Can you work these out from the model? Positions are in its coordinate system, mm. Round coordinates to 2 decimals unless told otherwise and drop trailing zeros. Write each loop counter-clockwise with the first axis right and the second up, starting at its lowest first coordinate (ties: lowest second). Pieces come first, ordered by that corner, then holes. Notation, with made-up numbers: M 22.5,66.25 L 59.5,66.25 A16 cw 59.5,91.25 Z; hole C -6,70 d11. An arc over 180 degrees is marked long. Answer as a JSON object with one key per item and string values. Group by question number.
1) Please list where these lines run through material, in increasing order: L1, parallel to X at y = 1.75, z = 54; L2, parallel to Z at x = 16, y = 1.6; L3, parallel to Z at x = -10.5, y = 0.4. Write a range as [from, to].
2) Suppose I cut it at A-A, the plane x = 24. State how many separate pieces and enclosed holes the cut face has, and give its area (3 significant figures).
3) I'm going to push flat-ended pins straight in: pin 1 Ø1 at (x, y) = (8, 0.5) entering from -Z; pin 2 Ø0.6 at (x, y) = (26, 0.5) entering from -Z; pin 3 Ø8 at (x, z) = (-10, 19) entering from -Y. Where does each tip first touch, or does it pass through?
4) Suppose I cut it at B-B, the plane z = 22. Write out the boundary of the cut face in (x, y).
from build123d import *

# Parameters (mm, degrees)
SKETCH2_W           = 105
SKETCH2_H           = 69
SKETCH2_W_2         = 12.176237233
SKETCH2_H_2         = 12
SKETCH2_W_3         = 12
SKETCH2_W_4         = 11
SKETCH2_H_3         = 11
SKETCH2_W_5         = 10.781198293
BOSS_EXTRUDE1_DEPTH = 2
FILLET1_R           = 5
FILLET2_R           = 5
CHAMFER1_SIZE       = 2
SKETCH3_W           = 12.4
SKETCH3_H           = 12.584292926
SKETCH3_W_2         = 12.5
SKETCH3_W_3         = 12.6
SKETCH3_W_4         = 12.2
SKETCH3_H_2         = 12.9
SKETCH3_H_3         = 12.6
CUT_EXTRUDE1_DEPTH  = 10
SKETCH4_W           = 0.6
SKETCH4_H           = 11
BOSS_EXTRUDE2_DEPTH = 2
SKETCH5_W           = 0.6
SKETCH5_H           = 11
BOSS_EXTRUDE3_DEPTH = 2
SKETCH6_W           = 0.8
SKETCH6_H           = 11
SKETCH6_W_2         = 0.4
SKETCH6_W_3         = 0.776237233
BOSS_EXTRUDE4_DEPTH = 2


with BuildPart() as part:
    # Sketch2 → Boss-Extrude1 (new body)
    with BuildSketch(Plane(origin=(0, 0, 0), x_dir=(1, 0, 0), z_dir=(0, 1, 0))):
        with Locations((0, -41.5)):
            Rectangle(SKETCH2_W, SKETCH2_H)
        with Locations((-23.611881384, -66)):
            Rectangle(SKETCH2_W_2, SKETCH2_H_2, mode=Mode.SUBTRACT)
        with Locations((11.3, -66)):
            Rectangle(SKETCH2_W_3, SKETCH2_H_2, mode=Mode.SUBTRACT)
        with Locations((28.8, -66)):
            Rectangle(SKETCH2_W_4, SKETCH2_H_2, mode=Mode.SUBTRACT)
        with Locations((28.8, -20.5)):
            Rectangle(SKETCH2_W_4, SKETCH2_H_3, mode=Mode.SUBTRACT)
        with Locations((11.3, -20.5)):
            Rectangle(SKETCH2_W_3, SKETCH2_H_3, mode=Mode.SUBTRACT)
        with Locations((-6.090599146, -20.5)):
            Rectangle(SKETCH2_W_5, SKETCH2_H_3, mode=Mode.SUBTRACT)
        with Locations((-6.090599146, -66)):
            Rectangle(SKETCH2_W_5, SKETCH2_H_2, mode=Mode.SUBTRACT)
        with Locations((-23.611881384, -20.5)):
            Rectangle(SKETCH2_W_2, SKETCH2_H_3, mode=Mode.SUBTRACT)
        with Locations((-23.611881384, -35.5)):
            Rectangle(SKETCH2_W_2, SKETCH2_H_3, mode=Mode.SUBTRACT)
        with Locations((-23.611881384, -50.5)):
            Rectangle(SKETCH2_W_2, SKETCH2_H_3, mode=Mode.SUBTRACT)
        with Locations((28.8, -50.5)):
            Rectangle(SKETCH2_W_4, SKETCH2_H_3, mode=Mode.SUBTRACT)
        with Locations((28.8, -35.5)):
            Rectangle(SKETCH2_W_4, SKETCH2_H_3, mode=Mode.SUBTRACT)
        with Locations((11.3, -50.5)):
            Rectangle(SKETCH2_W_3, SKETCH2_H_3, mode=Mode.SUBTRACT)
        with Locations((-6.090599146, -50.5)):
            Rectangle(SKETCH2_W_5, SKETCH2_H_3, mode=Mode.SUBTRACT)
        with Locations((-6.090599146, -35.5)):
            Rectangle(SKETCH2_W_5, SKETCH2_H_3, mode=Mode.SUBTRACT)
        with Locations((11.3, -35.5)):
            Rectangle(SKETCH2_W_3, SKETCH2_H_3, mode=Mode.SUBTRACT)
    extrude(amount=BOSS_EXTRUDE1_DEPTH)

    # Fillet1
    fillet1_edges = [part.edges().sort_by_distance(p)[0] for p in [
        (-52.5, 1, 76),
    ]]
    fillet(fillet1_edges, radius=FILLET1_R)

    # Fillet2
    fillet2_edges = [part.edges().sort_by_distance(p)[0] for p in [
        (52.5, 1, 76),
    ]]
    fillet(fillet2_edges, radius=FILLET2_R)

    # Chamfer1
    chamfer1_edges = [part.edges().sort_by_distance(p)[0] for p in [
        (0, 0, 7),
    ]]
    chamfer(chamfer1_edges, length=CHAMFER1_SIZE - 0.0001)  # a hair under: the kernel refuses the full size

    # Sketch3 → Cut-Extrude1 (cut)
    with BuildSketch(Plane(origin=(0, 2, 0), x_dir=(1, 0, 0), z_dir=(0, 1, 0))):
        with Locations((27.5, -20.492146463)):
            Rectangle(SKETCH3_W, SKETCH3_H)
        with Locations((10.25, -20.492146463)):
            Rectangle(SKETCH3_W_2, SKETCH3_H)
        with Locations((-7.4, -20.492146463)):
            Rectangle(SKETCH3_W_3, SKETCH3_H)
        with Locations((-24.4, -20.492146463)):
            Rectangle(SKETCH3_W_4, SKETCH3_H)
        Polygon((-30.5, -41.5), (-18.3, -41.5), (-18.3, -29.743553264), (-30.5, -29.683386914), align=None)
        Polygon((-13.7, -41.5), (-1.1, -41.5), (-1.1, -29.828377953), (-13.7, -29.766238937), align=None)
        Polygon((4, -41.5), (16.5, -41.5), (16.5, -29.91517531), (4, -29.85352946), align=None)
        Polygon((21.3, -41.5), (33.7, -41.5), (33.7, -30), (21.3, -29.938847317), align=None)
        with Locations((27.5, -50.65)):
            Rectangle(SKETCH3_W, SKETCH3_H_2)
        with Locations((10.25, -50.65)):
            Rectangle(SKETCH3_W_2, SKETCH3_H_2)
        with Locations((-7.4, -50.65)):
            Rectangle(SKETCH3_W_3, SKETCH3_H_2)
        with Locations((-24.4, -50.65)):
            Rectangle(SKETCH3_W_4, SKETCH3_H_2)
        with Locations((-24.4, -65.5)):
            Rectangle(SKETCH3_W_4, SKETCH3_H_3)
        with Locations((-7.4, -65.5)):
            Rectangle(SKETCH3_W_3, SKETCH3_H_3)
        with Locations((10.25, -65.5)):
            Rectangle(SKETCH3_W_2, SKETCH3_H_3)
        with Locations((27.5, -65.5)):
            Rectangle(SKETCH3_W, SKETCH3_H_3)
    extrude(amount=-CUT_EXTRUDE1_DEPTH, mode=Mode.SUBTRACT)

    # Sketch4 → Boss-Extrude2 (add)
    with BuildSketch(Plane(origin=(0, 2, 0), x_dir=(1, 0, 0), z_dir=(0, 1, 0))):
        with Locations((34, -20.5)):
            Rectangle(SKETCH4_W, SKETCH4_H)
    extrude(amount=-BOSS_EXTRUDE2_DEPTH)

    # Sketch5 → Boss-Extrude3 (add)
    with BuildSketch(Plane(origin=(0, 2, 0), x_dir=(1, 0, 0), z_dir=(0, 1, 0))):
        with Locations((34, -35.5)):
            Rectangle(SKETCH5_W, SKETCH5_H)
        with Locations((34, -50.5)):
            Rectangle(SKETCH5_W, SKETCH5_H)
        Polygon((33.7, -60), (34.3, -60), (34.3, -72), (23.3, -72), (23.3, -71.8), (33.7, -71.8), align=None)
    extrude(amount=-BOSS_EXTRUDE3_DEPTH)

    # Sketch6 → Boss-Extrude4 (add)
    with BuildSketch(Plane(origin=(0, 2, 0), x_dir=(1, 0, 0), z_dir=(0, 1, 0))):
        with Locations((16.9, -20.5)):
            Rectangle(SKETCH6_W, SKETCH6_H)
        with Locations((16.9, -35.5)):
            Rectangle(SKETCH6_W, SKETCH6_H)
        with Locations((16.9, -50.5)):
            Rectangle(SKETCH6_W, SKETCH6_H)
        Polygon((16.5, -60), (17.3, -60), (17.3, -72), (5.3, -72), (5.3, -71.8), (16.5, -71.8), align=None)
        Polygon((-1.1, -60), (-0.7, -60), (-0.7, -72), (-11.481198293, -72), (-11.481198293, -71.8), (-1.1, -71.8), align=None)
        Polygon((-18.3, -60), (-17.523762767, -60), (-17.523762767, -72), (-29.7, -72), (-29.7, -71.8), (-18.3, -71.8), align=None)
        with Locations((-0.9, -50.5)):
            Rectangle(SKETCH6_W_2, SKETCH6_H)
        with Locations((-0.9, -35.5)):
            Rectangle(SKETCH6_W_2, SKETCH6_H)
        with Locations((-0.9, -20.5)):
            Rectangle(SKETCH6_W_2, SKETCH6_H)
        with Locations((-17.911881384, -20.5)):
            Rectangle(SKETCH6_W_3, SKETCH6_H)
        with Locations((-17.911881384, -35.5)):
            Rectangle(SKETCH6_W_3, SKETCH6_H)
        with Locations((-17.911881384, -50.5)):
            Rectangle(SKETCH6_W_3, SKETCH6_H)
    extrude(amount=-BOSS_EXTRUDE4_DEPTH)


solid = part.part
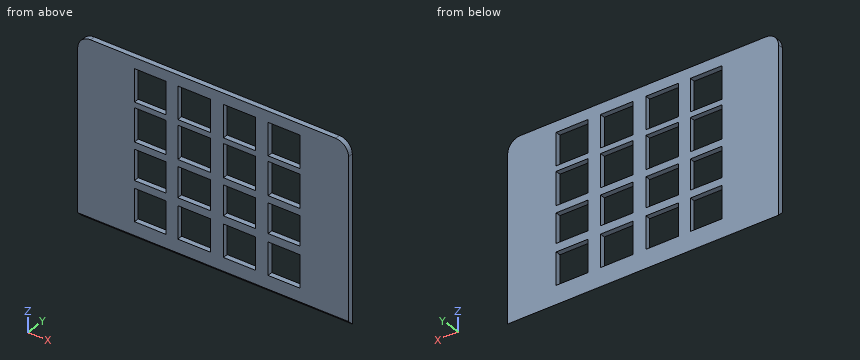
Results:
{
 "1": {"L1": "[-52.5, -30.5], [-18.3, -13.7], [-1.1, 4], [16.5, 21.3], [33.7, 52.5]", "L2": "[7.4, 14.2], [26.78, 29.91], [41.5, 44.2], [57.1, 59.2], [71.8, 76]", "L3": "[8.6, 14.2], [26.78, 29.78], [41.5, 44.2], [57.1, 59.2], [71.8, 76]"},
 "2": {"separate pieces": "5", "enclosed holes": "0", "area": "36.7 mm^2"},
 "3": {"pin 1": "z = 8", "pin 2": "z = 8.2", "pin 3": "y = 0"},
 "4": {"outline": "M -52.5,0 L -30.5,0 L -30.5,2 L -52.5,2 Z; M -18.3,0 L -13.7,0 L -13.7,2 L -18.3,2 Z; M -1.1,0 L 4,0 L 4,2 L -1.1,2 Z; M 16.5,0 L 21.3,0 L 21.3,2 L 16.5,2 Z; M 33.7,0 L 52.5,0 L 52.5,2 L 33.7,2 Z"}
}
